The model under review builds one solid part; all positions refer to its coordinate system, in mm. A direction names the side the tool comes from. Coordinates: 2 decimals unless noted, no trailing zeros. Order: outer loops, then holes, each group sorted by start corner. A loop starts at its lowest first (then second) coordinate and runs counter-clockwise, first axis right, second up. Notation, with made-up numbers: (-25.5, 78) - (-1.5, 78) arc R31 cw to (-1.5, 108) - close; hole circle Ø1 at (-33.75, 75.25). An arc over 180 degrees is marked (long way). Answer in a Markdown table with one row per item.
```python
from build123d import *

# Parameters (mm, degrees)
SKETCH1_W           = 0.65
SKETCH1_H           = 0.65
BOSS_EXTRUDE1_DEPTH = 8
BOSS_EXTRUDE2_DEPTH = 7


with BuildPart() as part:
    # Sketch1 → Boss-Extrude1 (new body)
    with BuildSketch(Plane.XY):
        Polygon((2.182384268, 30.912610308), (19.102384268, 30.912610308), (19.102384268, 29.912610308), (23.602384268, 29.912610308), (23.602384268, 30.912610308), (40.522384268, 30.912610308), (40.522384268, 37.912610308), (2.182384268, 37.912610308), align=None)
        with Locations((6.112384268, 33.142610308)):
            Rectangle(SKETCH1_W, SKETCH1_H, mode=Mode.SUBTRACT)
        with Locations((8.652384268, 33.142610308)):
            Rectangle(SKETCH1_W, SKETCH1_H, mode=Mode.SUBTRACT)
        with Locations((6.112384268, 35.682610308)):
            Rectangle(SKETCH1_W, SKETCH1_H, mode=Mode.SUBTRACT)
        with Locations((8.652384268, 35.682610308)):
            Rectangle(SKETCH1_W, SKETCH1_H, mode=Mode.SUBTRACT)
        with Locations((14.382384268, 33.142610308)):
            Rectangle(SKETCH1_W, SKETCH1_H, mode=Mode.SUBTRACT)
        with Locations((11.842384268, 35.682610308)):
            Rectangle(SKETCH1_W, SKETCH1_H, mode=Mode.SUBTRACT)
        with Locations((11.842384268, 33.142610308)):
            Rectangle(SKETCH1_W, SKETCH1_H, mode=Mode.SUBTRACT)
        with Locations((14.382384268, 35.682610308)):
            Rectangle(SKETCH1_W, SKETCH1_H, mode=Mode.SUBTRACT)
        with Locations((20.112384268, 33.142610308)):
            Rectangle(SKETCH1_W, SKETCH1_H, mode=Mode.SUBTRACT)
        with Locations((17.572384268, 35.682610308)):
            Rectangle(SKETCH1_W, SKETCH1_H, mode=Mode.SUBTRACT)
        with Locations((17.572384268, 33.142610308)):
            Rectangle(SKETCH1_W, SKETCH1_H, mode=Mode.SUBTRACT)
        with Locations((20.112384268, 35.682610308)):
            Rectangle(SKETCH1_W, SKETCH1_H, mode=Mode.SUBTRACT)
        with Locations((25.842384268, 33.142610308)):
            Rectangle(SKETCH1_W, SKETCH1_H, mode=Mode.SUBTRACT)
        with Locations((23.302384268, 35.682610308)):
            Rectangle(SKETCH1_W, SKETCH1_H, mode=Mode.SUBTRACT)
        with Locations((23.302384268, 33.142610308)):
            Rectangle(SKETCH1_W, SKETCH1_H, mode=Mode.SUBTRACT)
        with Locations((25.842384268, 35.682610308)):
            Rectangle(SKETCH1_W, SKETCH1_H, mode=Mode.SUBTRACT)
        with Locations((31.572384268, 33.142610308)):
            Rectangle(SKETCH1_W, SKETCH1_H, mode=Mode.SUBTRACT)
        with Locations((29.032384268, 35.682610308)):
            Rectangle(SKETCH1_W, SKETCH1_H, mode=Mode.SUBTRACT)
        with Locations((29.032384268, 33.142610308)):
            Rectangle(SKETCH1_W, SKETCH1_H, mode=Mode.SUBTRACT)
        with Locations((31.572384268, 35.682610308)):
            Rectangle(SKETCH1_W, SKETCH1_H, mode=Mode.SUBTRACT)
        with Locations((37.302384268, 33.142610308)):
            Rectangle(SKETCH1_W, SKETCH1_H, mode=Mode.SUBTRACT)
        with Locations((34.762384268, 35.682610308)):
            Rectangle(SKETCH1_W, SKETCH1_H, mode=Mode.SUBTRACT)
        with Locations((34.762384268, 33.142610308)):
            Rectangle(SKETCH1_W, SKETCH1_H, mode=Mode.SUBTRACT)
        with Locations((37.302384268, 35.682610308)):
            Rectangle(SKETCH1_W, SKETCH1_H, mode=Mode.SUBTRACT)
    extrude(amount=BOSS_EXTRUDE1_DEPTH)

    # Sketch2 → Boss-Extrude2 (add)
    with BuildSketch(Plane(origin=(0, 37.912610308, 0), x_dir=(1, 0, 0), z_dir=(0, 1, 0))):
        Polygon((3.429740031, 0), (3.429740031, 3), (39.275028505, 3), (39.275028505, 0), (37.775028505, 0), (37.775028505, 1.5), (4.929740031, 1.5), (4.929740031, 0), align=None)
    extrude(amount=-BOSS_EXTRUDE2_DEPTH)


solid = part.part
```
Item 1: We need section A-A, the plane y = 31.5. Write out the cut boundary in (x, z), then the cut area to 3 significant figures.
Check values:
| item | result |
|---|---|
| outline | (2.18, 0) - (3.43, 0) - (3.43, -3) - (39.28, -3) - (39.28, 0) - (40.52, 0) - (40.52, 8) - (2.18, 8) - close; hole (4.93, -1.5) - (37.78, -1.5) - (37.78, 0) - (4.93, 0) - close |
| area | 365 mm^2 |
Item 2: Tool access review of faces 1 (the face through (3.43, 34, -1)), 2 (the face through (4.93, 34, -1)), 3 (the face through (39.275, 34, -2)): name each direction out of +Z, -Z, +X, -X, +Y, -Y from which nothing blocks a thin tool from reaching the whole face with its end or side.
Check values:
| item | result |
|---|---|
| face 1 | -Z, -X, +Y, -Y |
| face 2 | +Y, -Y |
| face 3 | -Z, +X, +Y, -Y |
Item 3: We need section B-B, the plane x = 7. Write out the cut boundary in (y, z).
Check values:
| item | result |
|---|---|
| outline | (30.91, -3) - (37.91, -3) - (37.91, -1.5) - (30.91, -1.5) - close; (30.91, 0) - (37.91, 0) - (37.91, 8) - (30.91, 8) - close |
Item 4: We need section D-D, the plane x = 38.5. Write out the cut boundary in (y, z), then the cut area to 3 significant figures.
Check values:
| item | result |
|---|---|
| outline | (30.91, -3) - (37.91, -3) - (37.91, 8) - (30.91, 8) - close |
| area | 77.0 mm^2 |
Item 5: Mouldability with a two-part tool opening along Z and no side actions: class faces 4 (the face through (17, 30.913, 2)), 5 (the face through (40, 34, 0)), 6 (the face through (37.775, 34, -1)), 7 (the face through (21, 34, 8)) as +Z half, -Z half, draft (parallel to the pull), parting line (faces both ways), or undercut.
Check values:
| item | result |
|---|---|
| face 4 | draft |
| face 5 | -Z half |
| face 6 | undercut |
| face 7 | +Z half |
Item 6: Clearance check with a flat-ended pin moving along its axis: pin 1 Ø5 at (x, z) = (11, 7) entering from -Y. State where the tip first meets the part, or that it passes through.
Check values:
| item | result |
|---|---|
| pin 1 | y = 30.91 |
Item 7: We need section C-C, the plane z = 5. State how many separate pieces and enclosed holes the cut face has, then the cut area to 3 significant figures.
Check values:
| item | result |
|---|---|
| separate pieces | 1 |
| enclosed holes | 24 |
| area | 263 mm^2 |
Item 8: To check wall thickness, follow line 1 (X direction, y = 33.75, z = -0.5); line 2 (Z direction, x = 15, y = 35.25); line 3 (Y direction, x = 26, z = 0.5). State the ranges of each line that lie inside material, in increasing order. Write a range as from..to.
Check values:
| item | result |
|---|---|
| line 1 | 3.43..4.93, 37.78..39.28 |
| line 2 | -3..-1.5, 0..8 |
| line 3 | 30.91..32.82, 33.47..35.36, 36.01..37.91 |
